Geometry check sheet. Reference: the model listing, model coordinates, mm. Face numbers are marked on the shaded views. A direction names the side the tool comes from. Coordinates: 2 decimals unless noted, no trailing zeros. Loops run counter-clockwise (first coordinate to the right, second up) from the corner with the lowest first, then second, coordinate; pieces in that order, holes last. Notation, with made-up numbers: (-17, 32.5) - (34, 32.5) arc R7 cw to (34, 37.5) - close; hole circle Ø3 at (60.25, -23). An arc over 180 degrees is marked (long way). One line per item, written item: value.
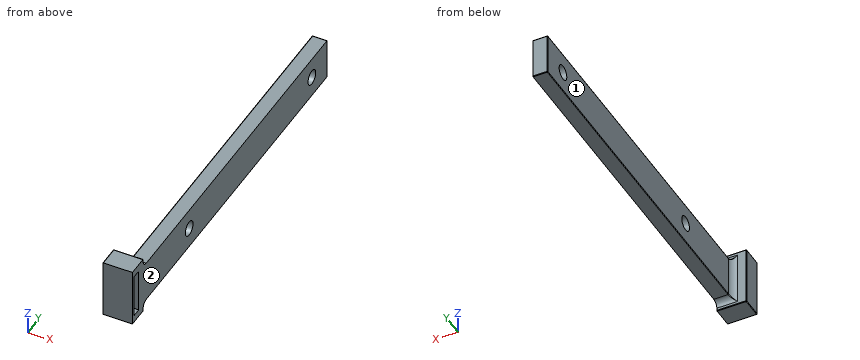
Autodesk Inventor part; units mm, degrees
ref_plane "YZ Plane" through (0, 0, 0) normal (1, 0, 0) x (0, 1, 0)
ref_plane "XZ Plane" through (0, 0, 0) normal (0, 1, 0) x (-1, 0, 0)
ref_plane "XY Plane" through (0, 0, 0) normal (0, 0, 1) x (1, 0, 0)
sketch "スケッチ1" plane through (0, 0, 0) normal (0, 1, 0) x (-1, 0, 0)
  line L0 (5, -10) -> (-5, -10)
  line L1 (-5, -10) -> (-5, 10)
  line L2 (-5, 10) -> (5, 10)
  line L3 (5, 10) -> (5, -10)
  line L4 (5, -10) -> (-5, 10) construction
  line L5 (-5, -10) -> (5, 10) construction
  point P0 (0, 0)
  dimension "d0" = 10
  dimension "d1" = 20
extrude "押し出し1" add sketch "スケッチ1" along normal blind 6
sketch "スケッチ2" plane through (0, 0, 0) normal (0, -1, 0) x (1, 0, 0)
  line L0 (5, 10) -> (5, -10)
  circle A0 centre (5, 0) radius 7.5
  point P0 (0, 0)
  point P1 (5, -7.5)
  point P2 (5, 7.5)
  dimension "d4" = 15
extrude "押し出し2" cut sketch "スケッチ2" against normal blind 3 contours L0 A0 picked at (1.9199, 0.374)
sketch "スケッチ3" plane through (0, 0, 0) normal (0, -1, 0) x (1, 0, 0)
  line L0 (-5, 10) -> (5, 10)
  line L1 (5, 10) -> (5, -10)
  line L2 (5, -10) -> (-5, -10)
  line L3 (-5, -10) -> (-5, 10)
  line L4 (-5, 10) -> (5, -10) construction
  line L5 (5, 10) -> (-5, -10) construction
  point P0 (0, 0)
  dimension "d7" = 10
  dimension "d8" = 20
extrude "押し出し3" add sketch "スケッチ3" along normal blind 1
sketch "スケッチ4" plane through (0, 6, 0) normal (0, 1, 0) x (1, 0, 0)
  line L0 (5, 7) -> (0, 7)
  line L1 (0, 7) -> (0, -7)
  line L2 (0, -7) -> (5, -7)
  line L3 (5, -7) -> (5, 7)
  line L4 (5, -10) -> (5, 10)
  point P0 (0, 0)
  dimension "d11" = 5
  dimension "d12" = 14
  dimension "d13" = 5
  dimension "d14" = 7
extrude "押し出し4" add sketch "スケッチ4" along normal blind 120
fillet "フィレット1" radius 2 3 edges at (2.5, 6, 7) (2.5, 6, -7) (0, 6, 0)
fillet "フィレット2" radius 0.2 12 edges at (-0.5858, 6.5858, -7.5858) (0, 67, -7) (-0.5858, 6.5858, 7.5858) (0, 67, 7) (2.5, 126, 7) (0, 126, 0) (2.5, 126, -7) (0, 6, -10) (-5, 6, 0) (0, 6, 10) (-5, 2.5, 10) (-5, 2.5, -10)
sketch "スケッチ5" plane through (0, 8, 6.8) normal (-1, 0, 0) x (0, 0, 1)
  line L0 (3, -2) -> (-16.6, -2)
  line L1 (-13.8, 117.8) -> (-13.8, 0)
  point P0 (-6.8, -8)
  point P1 (-6.8, 28)
  point P2 (-6.8, 108)
  dimension "d19" = 30
  dimension "d20" = 80
  dimension "d21" = 7
  dimension "d22" = 7
hole "穴1" at (0, 36, 0) at (0, 116, 0) direction (1, 0, 0) diameter 5 end through all
properties part number "baseB"
(1) Cross-section at A-A on y = 36. Record the cut outline in (x, z), and give its area (3 significant figures).
Reply:
outline: (0, -6.8) arc R0.2 ccw to (0.2, -7) - (5, -7) - (5, -2.5) - (0, -2.5) - close; (0, 2.5) - (5, 2.5) - (5, 7) - (0.2, 7) arc R0.2 ccw to (0, 6.8) - close
area: 45.0 mm2
(2) Material ranges on probe 1 along Y at (x, z) = (3.05, 0); probe 2 along Z at (x, y) = (1.95, 116); probe 3 along Y at (x, z) = (2.5, 0.75), recorded low to high. Write a range as from..to.
Reply:
probe 1: -1..0, 3..33.5, 38.5..113.5, 118.5..126
probe 2: -7..-2.5, 2.5..7
probe 3: -1..0, 3..33.62, 38.38..113.62, 118.38..126
(3) Access from +Z, -Z, +X, -X, +Y, -Y to the whole of each face (thin tool, end or side, straight path). Record for the marked faces 1 and 2.
Reply:
face 1: +Z, -Z, -X, +Y
face 2: +Z, -Z, +X, +Y, -Y
(4) Go/stop test with flat-tipped pins: pin 1 Ø3 at (y, z) = (73, -2) entering from -X; pin 2 Ø1.4 at (x, y) = (3.5, 87) entering from +Z; pin 3 Ø4 at (y, z) = (116, 0) entering from -X; pin 4 Ø5 at (x, y) = (-0.5, 104.5) entering from -Z. Record where each tip stops, or that it passes through.
Reply:
pin 1: x = 0
pin 2: z = 7
pin 3: through
pin 4: z = -7
(5) Cross-section at B-B on z = 0. Record the cut outline in (x, y).
Reply:
outline: (-5, -1) - (5, -1) - (5, 0) - (-2.5, 0) - (-2.5, 3) - (5, 3) - (5, 33.5) - (0, 33.5) - (0, 8) arc R2 cw to (-2, 6) - (-4.8, 6) arc R0.2 ccw to (-5, 5.8) - close; (0, 38.5) - (5, 38.5) - (5, 113.5) - (0, 113.5) - close; (0, 118.5) - (5, 118.5) - (5, 126) - (0.2, 126) arc R0.2 ccw to (0, 125.8) - close
(6) Cross-section at D-D on y = 57. Record the cut outline in (x, z), and give its area (3 significant figures).
Reply:
outline: (0, -6.8) arc R0.2 ccw to (0.2, -7) - (5, -7) - (5, 7) - (0.2, 7) arc R0.2 ccw to (0, 6.8) - close
area: 70.0 mm2
(7) Cross-section at C-C on x = 1.25. Record the cut outline in (y, z).
Reply:
outline: (-1, -10) - (5.8, -10) arc R0.2 ccw to (6, -9.8) - (6, -9) arc R2 cw to (8, -7) - (125.8, -7) arc R0.2 ccw to (126, -6.8) - (126, 6.8) arc R0.2 ccw to (125.8, 7) - (8, 7) arc R2 cw to (6, 9) - (6, 9.8) arc R0.2 ccw to (5.8, 10) - (-1, 10) - close; hole (0, -6.5) - (3, -6.5) - (3, 6.5) - (0, 6.5) - close; hole circle Ø5 at (36, 0); hole circle Ø5 at (116, 0)
